```python
from build123d import *

# Parameters (mm, degrees)
F0_W     = 40
F0_H     = 40
F1_DEPTH = 60
F2_W     = 50
F2_H     = 20
F3_DEPTH = 40.001
F4_R     = 5
F5_DEPTH = 25


with BuildPart() as f1:
    # F0 (on Right) → F1 (new body, symmetric)
    with BuildSketch(Plane.YZ):
        Rectangle(F0_W, F0_H)
    extrude(amount=F1_DEPTH, both=True)

    # F2 (on face) → F3 (cut, through all)
    with BuildSketch(Plane.XZ.offset(20)):
        with Locations((0, -10)):
            Rectangle(F2_W, F2_H)
    extrude(amount=-F3_DEPTH, mode=Mode.SUBTRACT)

    # F4 (on Right) → F5 (join, symmetric)
    with BuildSketch(Plane.YZ):
        with Locations((0, -10)):
            Circle(F4_R)
    extrude(amount=F5_DEPTH, both=True)


solid = f1.part
```
The listing builds one solid part. Answer for the finished solid, in the listing's coordinates (mm). A direction names the side the tool comes from. Coordinates: 2 decimals unless noted, no trailing zeros. Write each loop counter-clockwise with the first axis right and the second up, starting at its lowest first coordinate (ties: lowest second). Pieces come first, ordered by that corner, then holes.
Q1. Section B-B, the plane z = -3.5 is taken. Write down the section's boundary in (x, y).
Returned:
outline: (-60, -20) - (-25, -20) - (-25, 20) - (-60, 20) - close; (25, -20) - (60, -20) - (60, 20) - (25, 20) - close
Q2. The mould has two halves that part along X. Classify faces 1 (the cylindrical face through (0.35, -0.651, -5.043)), 2 (the flat face through (1, 0, 20)), 3 (the flat face through (60, 0, 0)): released by +X, released by -X, zero draft, split by the parting line, or undercut.
Returned:
face 1: undercut
face 2: zero draft
face 3: released by +X
Q3. Which of the six approach directions +Z, -Z, +X, -X, +Y, -Y give full straight-line access (tool end or side, diameter ignored) to faces 4 (the flat face through (0, 0, 0)), 5 (the flat face through (-60, 0, 0)), 6 (the flat face through (-25, -5, -8))?
Returned:
face 4: +Y, -Y
face 5: +Z, -Z, -X, +Y, -Y
face 6: none
Q4. Find the intervals of material crossed by line 1 along X through (y, z) = (-18, -13); line 2 along Z through (x, y) = (-17, 14.5); line 3 along Z through (x, y) = (-9, -3), in increasing order.
Returned:
line 1: x = -60 to -25, 25 to 60
line 2: z = 0 to 20
line 3: z = -14 to -6, 0 to 20
Q5. Section C-C, the plane x = 20 is taken. Write down the section's boundary in (y, z), then the cut area to 3 significant figures.
Returned:
outline: (-20, 0) - (20, 0) - (20, 20) - (-20, 20) - close; circle Ø10 at (0, -10)
area: 879 mm2
Q6. Given P1, Ø2, axis at x = -21.5, y = -1, coming from the -Z side; P2, Ø12, axis at x = -7.5, y = 10, coming from the -Z side, each flat-ended and moving along its own axis, determine where each tip first touches the part or whether it passes through.
Returned:
P1: stops at z = -15
P2: stops at z = -13
Q7. Section A-A, the plane y = 0 is taken. Write down the section's boundary in (x, z).
Returned:
outline: (-60, -20) - (-25, -20) - (-25, -15) - (25, -15) - (25, -20) - (60, -20) - (60, 20) - (-60, 20) - close; hole (-25, -5) - (25, -5) - (25, 0) - (-25, 0) - close
Q8. Section D-D, the plane z = -10 is taken. Write down the section's boundary in (x, y).
Returned:
outline: (-60, -20) - (-25, -20) - (-25, -5) - (25, -5) - (25, -20) - (60, -20) - (60, 20) - (25, 20) - (25, 5) - (-25, 5) - (-25, 20) - (-60, 20) - close
